Can you work these out from the drawing? Everything is in mm from the part's minimum corner. A direction names the side the tool comes from. Round coordinates to 2 decimals unless told otherwise and drop trailing zeros. Loops run counter-clockwise (first coordinate to the right, second up) from the corner with the lowest first, then second, coordinate; pieces in that order, holes last. Notation, with made-up numbers: (42, 39) - (62, 39) arc R22 ccw to (62, 73) - close; hole circle Ø1 at (85.25, 80). An arc over 180 degrees is marked (long way). Answer as a JSON object with one key per item and string values. Group by question number.
1) Will these pins go through, and if not, where does the flat tip stop? P1, Ø1.3, axis at x = 2, y = 21.8, coming from the +Z side; P2, Ø3, axis at x = 23, y = 9.3, coming from the +Z side; P3, Ø1.6, axis at x = 14.5, z = 2.5, coming from the +Y side.
2) I want a section at B-B, the plane y = 9.3. Please give me the cut outline in (x, z), then the cut area to 3 significant figures.
3) Which directions (+Z, -Z, +X, -X, +Y, -Y) give clear straight access to the entire face, cutting with the end or side of a thin tool? Please do the marked faces 1 and 2.
4) If we mould it in two halves opening along X, with no side actions, what happens to the marked faces 3, 4 and 5? For each: pulls with the +X half, pulls with the -X half, needs draft (parallel to the pull), parting line crosses it, or undercut.
5) I want a section at A-A, the plane y = 14.75. Please give me the cut outline in (x, z).
6) I want a section at C-C, the plane x = 23.5. Please give me the cut outline in (y, z).
7) I want a section at D-D, the plane z = 0.6. Please give me the cut outline in (x, y).
8) If I drill on line 1 along Y through (x, z) = (23, 0.95); line 2 along X through (y, z) = (11.75, 2.15); line 3 along X through (y, z) = (9.3, 2.55), over which ranges is the centre line in solid material (lowest first)? Write a range as [from, to].
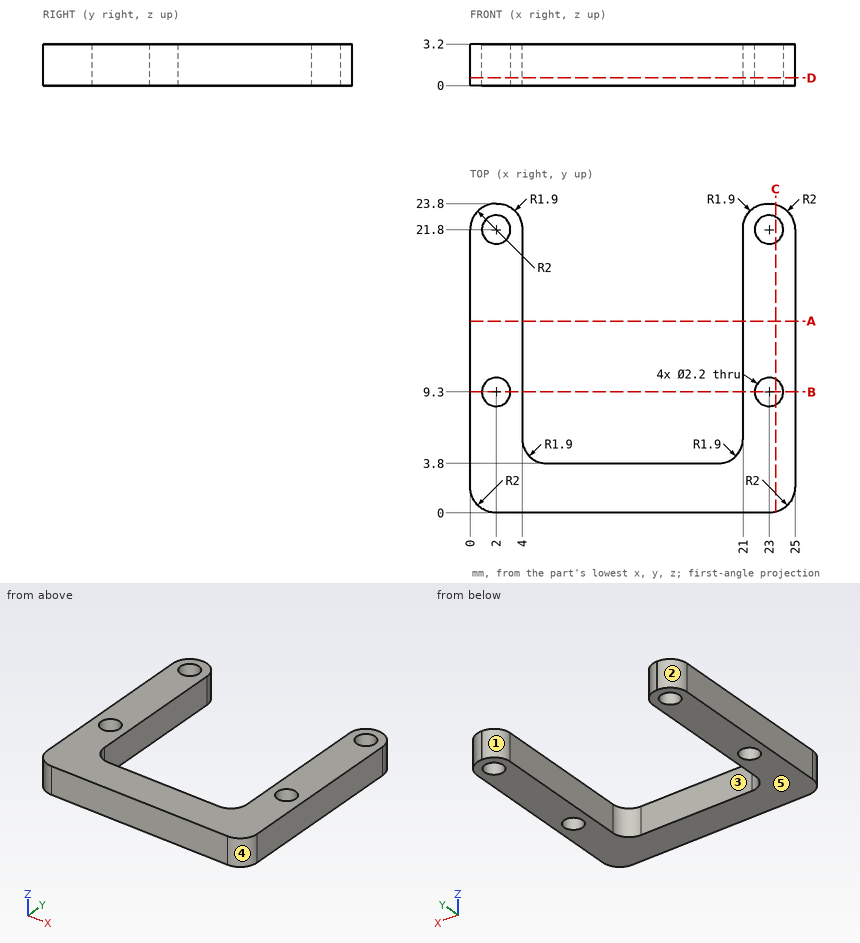
Outcome:
{
 "1": {"P1": "through", "P2": "z = 3.2", "P3": "y = 3.8"},
 "2": {"outline": "(0, 0) - (0.9, 0) - (0.9, 3.2) - (0, 3.2) - close; (3.1, 0) - (4, 0) - (4, 3.2) - (3.1, 3.2) - close; (21, 0) - (21.9, 0) - (21.9, 3.2) - (21, 3.2) - close; (24.1, 0) - (25, 0) - (25, 3.2) - (24.1, 3.2) - close", "area": "11.5 mm^2"},
 "3": {"face 1": "+Z, -Z, +Y", "face 2": "+Z, -Z, -X, +Y"},
 "4": {"face 3": "undercut", "face 4": "pulls with the +X half", "face 5": "needs draft"},
 "5": {"outline": "(0, 0) - (4, 0) - (4, 3.2) - (0, 3.2) - close; (21, 0) - (25, 0) - (25, 3.2) - (21, 3.2) - close"},
 "6": {"outline": "(0.06, 0) - (8.32, 0) - (8.32, 3.2) - (0.06, 3.2) - close; (10.28, 0) - (20.82, 0) - (20.82, 3.2) - (10.28, 3.2) - close; (22.78, 0) - (23.74, 0) - (23.74, 3.2) - (22.78, 3.2) - close"},
 "7": {"outline": "(0, 2) arc R2 ccw to (2, 0) - (23, 0) arc R2 ccw to (25, 2) - (25, 21.8) arc R2 ccw to (23, 23.8) - (22.9, 23.8) arc R1.9 ccw to (21, 21.9) - (21, 5.7) arc R1.9 cw to (19.1, 3.8) - (5.9, 3.8) arc R1.9 cw to (4, 5.7) - (4, 21.9) arc R1.9 ccw to (2.1, 23.8) - (2, 23.8) arc R2 ccw to (0, 21.8) - close; hole circle Ø2.2 at (2, 9.3); hole circle Ø2.2 at (2, 21.8); hole circle Ø2.2 at (23, 9.3); hole circle Ø2.2 at (23, 21.8)"},
 "8": {"line 1": "[0, 8.2], [10.4, 20.7], [22.9, 23.8]", "line 2": "[0, 4], [21, 25]", "line 3": "[0, 0.9], [3.1, 4], [21, 21.9], [24.1, 25]"}
}
